Part model, mm, in its own coordinate system. Face numbers are marked on the shaded views. A direction names the side the tool comes from. Round coordinates to 2 decimals unless told otherwise and drop trailing zeros. Loops run counter-clockwise (first coordinate to the right, second up) from the corner with the lowest first, then second, coordinate; pieces in that order, holes last.
from build123d import *

# Parameters (mm, degrees)
BOSS_EXTRUDE1_DEPTH = 22
FILLET1_R           = 10
SKETCH2_R           = 1.725
CUT_EXTRUDE1_DEPTH  = 132.244047484
SKETCH3_R           = 2.8
CUT_EXTRUDE2_DEPTH  = 119
FILLET2_R           = 10
CHAMFER1_SIZE       = 1


with BuildPart() as part:
    # Sketch1 → Boss-Extrude1 (new body)
    with BuildSketch(Plane.XY):
        Polygon((-64.5, 10), (64.5, 10), (64.5, -10), (59.5, -10), (59.5, 5), (-59.5, 5), (-59.5, -10), (-64.5, -10), align=None)
    extrude(amount=BOSS_EXTRUDE1_DEPTH)

    # Fillet1
    fillet1_edges = [part.edges().sort_by_distance(p)[0] for p in [
        (-59.5, 5, 11),
        (59.5, 5, 11),
    ]]
    fillet(fillet1_edges, radius=FILLET1_R)

    # Sketch2 → Cut-Extrude1 (cut, through all)
    with BuildSketch(Plane(origin=(64.5, 0, 0), x_dir=(0, 0, -1), z_dir=(1, 0, 0))):
        with Locations((-10, -2.5)):
            Circle(SKETCH2_R)
    extrude(amount=-CUT_EXTRUDE1_DEPTH, mode=Mode.SUBTRACT)

    # Sketch3 → Cut-Extrude2 (cut)
    with BuildSketch(Plane.ZY.offset(-59.5)):
        with Locations((10, -2.5)):
            Circle(SKETCH3_R)
    extrude(amount=CUT_EXTRUDE2_DEPTH, mode=Mode.SUBTRACT)

    # Fillet2
    # the kernel refuses this fillet: 10 mm, written as the material it takes off along each edge
    with BuildSketch(Plane(origin=(89.5, -10, 22), x_dir=(0, 1, 0), z_dir=(-1, 0, 0))) as fillet2_piece_1:
        with BuildLine():
            CenterArc((FILLET2_R, FILLET2_R), FILLET2_R, 180, 90)
            Line((0, FILLET2_R), (0, 0))
            Line((0, 0), (FILLET2_R, 0))
        make_face()
    extrude(amount=55, mode=Mode.SUBTRACT)
    with BuildSketch(Plane(origin=(-34.5, -10, 22), x_dir=(0, 0, -1), z_dir=(-1, 0, 0))) as fillet2_piece_2:
        with BuildLine():
            CenterArc((FILLET2_R, -FILLET2_R), FILLET2_R, 90, 90)
            Line((0, -FILLET2_R), (0, 0))
            Line((0, 0), (FILLET2_R, 0))
        make_face()
    extrude(amount=55, mode=Mode.SUBTRACT)

    # Chamfer1
    chamfer1_edges = [part.edges().sort_by_distance(p)[0] for p in [
        (62, -10, 0),
        (-62, -10, 0),
    ]]
    chamfer(chamfer1_edges, length=CHAMFER1_SIZE)


solid = part.part
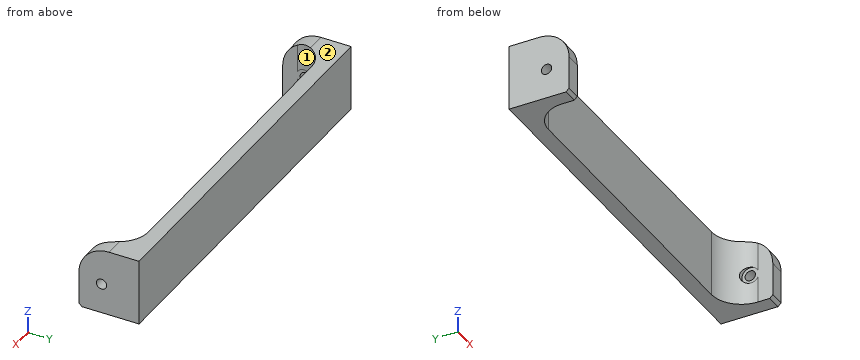
1) Slice it at C-C, the plane y = -2.5. Give the cut face in (x, z) (3 decimals), then the cut area to 3 significant figures.
Values:
outline: (-64.5, 0) - (-59.182, 0) - (-59.182, 7.2) - (-59.5, 7.2) - (-59.5, 8.275) - (-64.5, 8.275) - close; (-64.5, 11.725) - (-59.5, 11.725) - (-59.5, 12.8) - (-59.182, 12.8) - (-59.182, 21.682) - (-64.5, 21.682) - close; (59.182, 0) - (64.5, 0) - (64.5, 8.275) - (59.5, 8.275) - (59.5, 7.2) - (59.182, 7.2) - close; (59.182, 12.8) - (59.5, 12.8) - (59.5, 11.725) - (64.5, 11.725) - (64.5, 21.682) - (59.182, 21.682) - close
area: 193 mm2
2) Slice it at D-D, the plane x = 34. Give the cut face in (y, z).
Values:
outline: (5, 0) - (10, 0) - (10, 22) - (5, 22) - close
3) Slice it at A-A, the plane z = 10. Give the cut face in (x, y) (3 decimals), then the cut area to 3 significant figures.
Values:
outline: (-64.5, -10) - (-59.5, -10) - (-59.5, -4.225) - (-64.5, -4.225) - close; (-64.5, -0.775) - (-59.5, -0.775) - (-59.5, 0.3) - (-57.98, 0.3) arc R10 cw to (-49.5, 5) - (49.5, 5) arc R10 cw to (57.98, 0.3) - (59.5, 0.3) - (59.5, -0.775) - (64.5, -0.775) - (64.5, 10) - (-64.5, 10) - close; (59.5, -10) - (64.5, -10) - (64.5, -4.225) - (59.5, -4.225) - close
area: 798 mm2
4) Slice it at B-B, the plane y = 3. Give the cut face in (x, z), then the cut area to 3 significant figures.
Values:
outline: (-64.5, 0) - (-55.5, 0) - (-55.5, 22) - (-64.5, 22) - close; (55.5, 0) - (64.5, 0) - (64.5, 22) - (55.5, 22) - close
area: 396 mm2
5) Wall check: line 1 along Y through (x, z) = (-62.3, 10) (3 decimals); line 2 along X through (y, z) = (-1.5, 7.75); line 3 along Y through (x, z) = (-32, 19.25). Give the ranges that are in metal, low to high.
Values:
line 1: y = -10 to -4.225, -0.775 to 10
line 2: x = -64.5 to -59.5, 59.5 to 64.5
line 3: y = 5 to 10
6) Drop flat-ended pins along their axis: pin 1 Ø5 at (x, z) = (14.5, 9.5) entering from -Y; pin 2 Ø12 at (x, y) = (2.5, -6) entering from -Z. Give the stop position or say it passes through.
Values:
pin 1: stops at y = 5
pin 2: passes through
7) Tool access for the marked faces 1 and 2: list every direction of +Z, -Z, +X, -X, +Y, -Y with a clear straight run to the whole face (end or side of a thin tool).
Values:
face 1: +Z, -Z, -Y
face 2: +Z, +X, -X, +Y, -Y
